Verification items for the finished model (mm, model axes). Coordinates: 2 decimals unless noted, no trailing zeros. Write each loop counter-clockwise with the first axis right and the second up, starting at its lowest first coordinate (ties: lowest second). Pieces come first, ordered by that corner, then holes. Notation, with made-up numbers: (-12.75, 69) - (7.25, 69) arc R17 ccw to (7.25, 92) - close; hole circle Ø11 at (7.25, 32). An arc over 180 degrees is marked (long way). Use one line per item in the form item = value. Start each with the question number.
(1) Sectioned sample at B-B (y = 0). Record the cut outline in (x, z), and give its area (3 significant figures).
(2) Gauge pin test, flat ends, axial feed: pin 1 Ø0.6 at (x, y) = (-21, 0) entering from +Z; pin 2 Ø0.6 at (x, z) = (27.5, 2) entering from -Y; pin 3 Ø1.5 at (x, y) = (-5.5, -1.5) entering from -Z; pin 4 Ø1 at (x, y) = (30.5, 0) entering from -Z. Record the tip position at first contact, or that the pin passes through.
(3) Sectioned sample at D-D (y = 5.75). Record the cut outline in (x, z), and give its area (3 significant figures).
(4) Material ranges on line 1 (X direction, y = -0.25, z = 4.35); line 2 (Y direction, x = -10, z = 2.3); line 3 (X direction, y = -1, z = 0.35), recorded low to high. Write a range as [from, to].
(5) Sectioned sample at A-A (z = 2.6). Record the cut outline in (x, y), and give its area (3 significant figures).
(6) Sectioned sample at C-C (x = -31). Record the cut outline in (y, z).
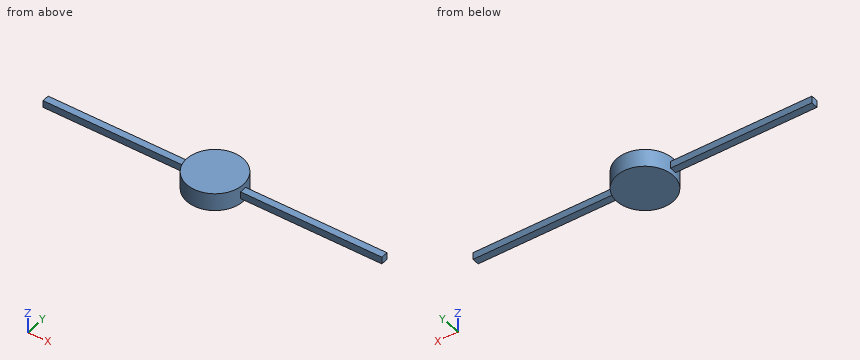
from build123d import *

# Parameters (mm, degrees)
SKETCH1_R           = 8
BOSS_EXTRUDE1_DEPTH = 5
SKETCH2_W           = 2
SKETCH2_H           = 2
BOSS_EXTRUDE2_DEPTH = 48


with BuildPart() as part:
    # Sketch1 → Boss-Extrude1 (new body)
    with BuildSketch(Plane.XY):
        Circle(SKETCH1_R)
    extrude(amount=BOSS_EXTRUDE1_DEPTH)

    # Sketch2 → Boss-Extrude2 (add)
    with BuildSketch(Plane.ZY.offset(48)):
        with Locations((2.5, 0)):
            Rectangle(SKETCH2_W, SKETCH2_H)
    boss_extrude2 = extrude(amount=-BOSS_EXTRUDE2_DEPTH)

    # Mirror1: Boss-Extrude2 across plane
    add(boss_extrude2.mirror(Plane(origin=(0, 0, 0), x_dir=(0, 0, 1), z_dir=(1, 0, 0))))


solid = part.part
Answers below:
q1.outline = (-48, 1.5) - (-8, 1.5) - (-8, 0) - (8, 0) - (8, 1.5) - (48, 1.5) - (48, 3.5) - (8, 3.5) - (8, 5) - (-8, 5) - (-8, 3.5) - (-48, 3.5) - close
q1.area = 240 mm2
q2.pin_1 = 3.5
q2.pin_2 = -1
q2.pin_3 = 0
q2.pin_4 = 1.5
q3.outline = (-5.56, 0) - (5.56, 0) - (5.56, 5) - (-5.56, 5) - close
q3.area = 55.6 mm2
q4.line_1 = [-8, 8]
q4.line_2 = [-1, 1]
q4.line_3 = [-7.94, 7.94]
q5.outline = (-48, -1) - (-7.94, -1) arc R8 ccw to (7.94, -1) - (48, -1) - (48, 1) - (7.94, 1) arc R8 ccw to (-7.94, 1) - (-48, 1) - close
q5.area = 361 mm2
q6.outline = (-1, 1.5) - (1, 1.5) - (1, 3.5) - (-1, 3.5) - close
